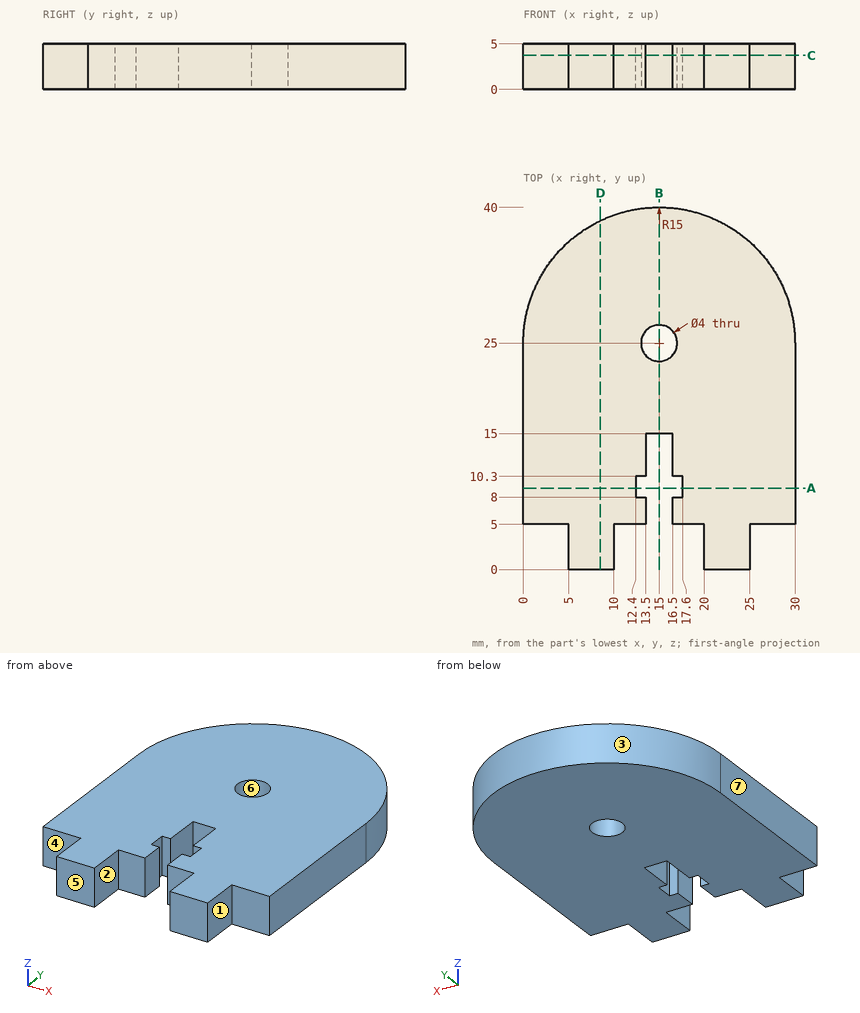
Here's the drawing with two shaded views (mm, measured from the low corner). I have some questions. A direction names the side the tool comes from. Give positions to 0.01 mm unless a question says otherwise; leave off trailing zeros. Loops run counter-clockwise (first coordinate to the right, second up) from the corner with the lowest first, then second, coordinate; pieces in that order, holes last. Notation, with made-up numbers: (80, 82) -> (137, 82) arc R32 cw to (137, 113) -> close; hole circle Ø10 at (1, 69). An arc over 180 degrees is marked (long way). Answer as a JSON object with one key per item and string values. Group by question number.
Item 1: Imagine slicing it at C-C on z = 3.75. Write out the boundary of the cut face in (x, y).
Item 2: Will these pins go through, and if not, where does the flat tip stop? pin 1 (2.5 mm diameter, centred on x = 15.5, z = 2, fed in from -Y); pin 2 (1.8 mm diameter, centred on y = 9, z = 3, fed in from -X); pin 3 (3 mm diameter, centred on x = 15, y = 4.5, fed in from -Z); pin 4 (0.9 mm diameter, centred on x = 17, z = 2, fed in from +Y).
Item 3: Imagine slicing it at D-D on x = 8.5. Write out the boundary of the cut face in (y, z).
Item 4: I need wall thicknesses on L1, parallel to X at y = 9, z = 2.8; L2, parallel to X at y = 7.5, z = 4.35; L3, parallel to Y at x = 15, z = 3.3. Which ranges of each line are inside material? Lowest first, please.
Item 5: Imagine slicing it at B-B on x = 15. Write out the boundary of the cut face in (y, z), then the cut area to 3 significant figures.
Item 6: Imagine slicing it at A-A on y = 9. Write out the boundary of the cut face in (x, z), then the cut area to 3 significant figures.
Item 7: Thinking about a two-plate mould opening in Y: for the marked faces 5, 6 and 7, which applies, pulls with the +Y half, pulls with the -Y half, needs draft (parallel to the pull), parting line crosses it, or undercut?
Item 8: On a 3-axis mill with a long thin cutter (end or side, diameter ignored), from which of +Z, -Z, +X, -X, +Y, -Y can I reach the whole of each face in a straight line? I mean the marked faces 1, 2, 3 and 4. Say none if no direction works.
Answer list:
{
 "1": {"outline": "(0, 5) -> (5, 5) -> (5, 0) -> (10, 0) -> (10, 5) -> (13.5, 5) -> (13.5, 8) -> (12.4, 8) -> (12.4, 10.3) -> (13.5, 10.3) -> (13.5, 15) -> (16.5, 15) -> (16.5, 10.3) -> (17.6, 10.3) -> (17.6, 8) -> (16.5, 8) -> (16.5, 5) -> (20, 5) -> (20, 0) -> (25, 0) -> (25, 5) -> (30, 5) -> (30, 25) arc R15 ccw to (0, 25) -> close; hole circle Ø4 at (15, 25)"},
 "2": {"pin 1": "stops at y = 5", "pin 2": "stops at x = 0", "pin 3": "passes through", "pin 4": "stops at y = 39.92"},
 "3": {"outline": "(0, 0) -> (38.52, 0) -> (38.52, 5) -> (0, 5) -> close"},
 "4": {"L1": "x = 0 to 12.4, 17.6 to 30", "L2": "x = 0 to 13.5, 16.5 to 30", "L3": "y = 15 to 23, 27 to 40"},
 "5": {"outline": "(15, 0) -> (23, 0) -> (23, 5) -> (15, 5) -> close; (27, 0) -> (40, 0) -> (40, 5) -> (27, 5) -> close", "area": "105 mm2"},
 "6": {"outline": "(0, 0) -> (12.4, 0) -> (12.4, 5) -> (0, 5) -> close; (17.6, 0) -> (30, 0) -> (30, 5) -> (17.6, 5) -> close", "area": "124 mm2"},
 "7": {"face 5": "pulls with the -Y half", "face 6": "undercut", "face 7": "needs draft"},
 "8": {"face 1": "+Z, -Z, +X, -Y", "face 2": "+Z, -Z, -Y", "face 3": "+Z, -Z, +Y", "face 4": "+Z, -Z, -X, -Y"}
}
